Can you work these out from the model? Positions are in its coordinate system, mm. Give positions to 0.01 mm unless a question says otherwise; leave off trailing zeros. Order: outer loops, then holes, each group sorted by start corner. A loop starts at its lowest first (then second) coordinate and runs counter-clockwise, first axis right, second up. Notation, with made-up numbers: M -13,18 L 22,18 A20 cw 22,32 Z; hole C 62,42.25 d10. An arc over 180 degrees is marked long. Write each question's results on one line, items separated by ' | '.
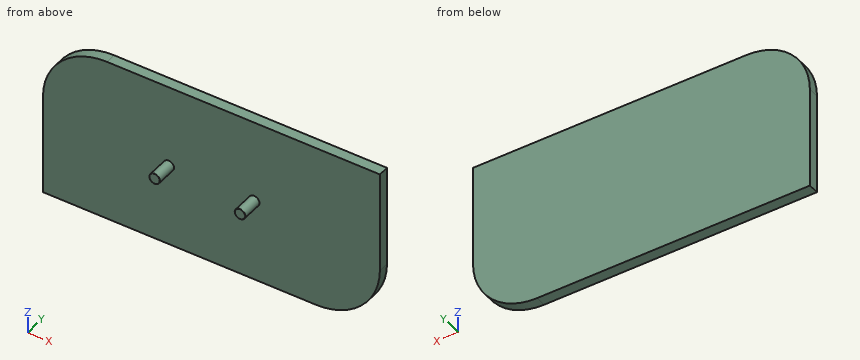
from build123d import *

# Parameters (mm, degrees)
F1_DEPTH = 5
F2_R     = 2.5
F3_DEPTH = 10
F4_R     = 0.2


with BuildPart() as f1:
    # F0 (on Front) → F1 (new body)
    with BuildSketch(Plane.XZ):
        with BuildLine():
            Line((78.891635, -8.808454), (78.891635, 38.808454))
            Line((78.891635, 38.808454), (-48.891635, 38.808454))
            ThreePointArc((-48.891635, 38.808454), (-70.104838, 30.021657), (-78.891635, 8.808454))
            Line((-78.891635, 8.808454), (-78.891635, -38.808454))
            Line((-78.891635, -38.808454), (48.891635, -38.808454))
            ThreePointArc((48.891635, -38.808454), (70.104838, -30.021657), (78.891635, -8.808454))
        make_face()
    extrude(amount=F1_DEPTH)

    # F2 (on face) → F3 (join)
    with BuildSketch(Plane.XZ.offset(5)):
        with Locations((-20, 0)):
            Circle(F2_R)
        with Locations((20, 0)):
            Circle(F2_R)
    extrude(amount=F3_DEPTH)

    # F4
    f4_edges = [f1.edges().sort_by_distance(p)[0] for p in [
        (-22.5, -15, 0),
        (17.5, -15, 0),
    ]]
    fillet(f4_edges, radius=F4_R)


solid = f1.part
(1) Imagine slicing it at B-B, the plane x = 20. Write out the boundary of the cut face in (y, z).
Data:
outline: M -15,-2.3 A0.2 ccw -14.8,-2.5 L -5,-2.5 L -5,-38.81 L 0,-38.81 L 0,38.81 L -5,38.81 L -5,2.5 L -14.8,2.5 A0.2 ccw -15,2.3 Z
(2) Will these pins go through, and if not, where does the flat tip stop? P1, Ø1, axis at x = 13, y = -6, coming from the +Z side; P2, Ø6, axis at y = -3.5, z = -12, coming from the +X side; P3, Ø6, axis at x = -52.5, z = 3, coming from the -Y side.
Data:
P1: passes through | P2: stops at x = 78.89 | P3: stops at y = -5
(3) Imagine slicing it at D-D, the plane x = -4. Write out the boundary of the cut face in (y, z).
Data:
outline: M -5,-38.81 L 0,-38.81 L 0,38.81 L -5,38.81 Z
(4) Imagine slicing it at C-C, the plane z = 0. Write out the boundary of the cut face in (x, y).
Data:
outline: M -78.89,-5 L -22.5,-5 L -22.5,-14.8 A0.2 ccw -22.3,-15 L -17.7,-15 A0.2 ccw -17.5,-14.8 L -17.5,-5 L 17.5,-5 L 17.5,-14.8 A0.2 ccw 17.7,-15 L 22.3,-15 A0.2 ccw 22.5,-14.8 L 22.5,-5 L 78.89,-5 L 78.89,0 L -78.89,0 Z
(5) I need wall thicknesses on L1, parallel to Y at x = -7.5, z = 31; L2, parallel to Z at x = 52.5, y = -1.5; L3, parallel to Z at x = 65, y = -3.75. Which ranges of each line are inside material? Lowest first, please. Write a range as from..to.
Data:
L1: y = -5..0 | L2: z = -38.59..38.81 | L3: z = -34.12..38.81
(6) Imagine slicing it at A-A, the plane y = -9.25. Write out the boundary of the cut face in (x, z), plus the area to 3 significant figures.
Data:
outline: C -20,0 d5; C 20,0 d5 | area: 39.3 mm2
